```python
from build123d import *
from OCP.BRepFilletAPI import BRepFilletAPI_MakeChamfer

# Parameters (mm, degrees)
SKETCH_1_W          = 23
SKETCH_1_H          = 2
EXTRUDE_1_DEPTH     = 5
CHAMFER_1_SIZE      = 2
CHAMFER_1_SIZE2     = 1.678199262
SKETCH_2_W          = 5
SKETCH_2_H          = 2
EXTRUDE_2_DEPTH     = 14
CUT_EXTRUDE_1_DEPTH = 27.944387171
SKETCH_4_W          = 5
SKETCH_4_H          = 2
EXTRUDE_3_DEPTH     = 0.5
CHAMFER_3_SIZE      = 0.419549816
CHAMFER_3_SIZE_2    = 0.5
SKETCH_5_W          = 5
SKETCH_5_H          = 2
CUT_EXTRUDE_2_DEPTH = 19.227726134
CHAMFER_4_SIZE      = 1.5
CHAMFER_4_SIZE2     = 0.545955351
SKETCH_6_W          = 5
SKETCH_6_H          = 2
EXTRUDE_4_DEPTH     = 0.5
CHAMFER_5_SIZE      = 0.5
CHAMFER_6_SIZE      = 0.5
CHAMFER_6_SIZE2     = 1.37373871


with BuildPart() as part:
    # 草图1 → 凸台-拉伸1 (new body)
    with BuildSketch(Plane(origin=(0, 0, 0), x_dir=(1, 0, 0), z_dir=(0, 1, 0))):
        Rectangle(SKETCH_1_W, SKETCH_1_H)
    extrude(amount=EXTRUDE_1_DEPTH)

    # 倒角1
    chamfer_1_edges = [part.edges().sort_by_distance(p)[0] for p in [
        (0, 5, 1),
    ]]
    chamfer_1_side = [part.faces().sort_by_distance(p)[0] for p in [
        (0, 2.5, 1),
    ]]
    chamfer(chamfer_1_edges, length=CHAMFER_1_SIZE, length2=CHAMFER_1_SIZE2, reference=chamfer_1_side[0])

    # 草图2 → 凸台-拉伸2 (add)
    with BuildSketch(Plane(origin=(0, 0, 0), x_dir=(1, 0, 0), z_dir=(0, 1, 0))):
        with Locations((-9, 0)):
            Rectangle(SKETCH_2_W, SKETCH_2_H)
        with Locations((9, 0)):
            Rectangle(SKETCH_2_W, SKETCH_2_H)
    extrude(amount=EXTRUDE_2_DEPTH)

    # 草图3 → 切除-拉伸1 (cut, through all)
    with BuildSketch(Plane(origin=(11.5, 0, 0), x_dir=(0, 0, -1), z_dir=(1, 0, 0))):
        Polygon((-1, 1.821800738), (1, 3.5), (1, 0), (-1, 0), align=None)
    extrude(amount=-CUT_EXTRUDE_1_DEPTH, mode=Mode.SUBTRACT)

    # 草图4 → 凸台-拉伸3 (add)
    with BuildSketch(Plane(origin=(0, 0, -1), x_dir=(-1, 0, 0), z_dir=(0, 0, -1))):
        with Locations((-9, 13)):
            Rectangle(SKETCH_4_W, SKETCH_4_H)
    extrude(amount=EXTRUDE_3_DEPTH)

    # 倒角3
    chamfer_3_edges_1 = [part.edges().sort_by_distance(p)[0] for p in [
        (9, 12, -1.5),
    ]]
    chamfer_3_side_1 = [part.faces().sort_by_distance(p)[0] for p in [
        (9, 12.008390996, -1.5),
    ]]
    chamfer_3_edges_2 = [part.edges().sort_by_distance(p)[0] for p in [
        (9, 14, -1.5),
    ]]
    chamfer_3_side_2 = [part.faces().sort_by_distance(p)[0] for p in [
        (9, 13.991609004, -1.5),
    ]]
    chamfer_3 = BRepFilletAPI_MakeChamfer(part.part.solid().wrapped)
    for e in chamfer_3_edges_1:
        chamfer_3.Add(CHAMFER_3_SIZE - 0.0001, CHAMFER_3_SIZE_2 - 0.0001, e.wrapped, chamfer_3_side_1[0].wrapped)
    for e in chamfer_3_edges_2:
        chamfer_3.Add(CHAMFER_3_SIZE - 0.0001, CHAMFER_3_SIZE_2 - 0.0001, e.wrapped, chamfer_3_side_2[0].wrapped)
    add(Compound.cast(chamfer_3.Shape()), mode=Mode.REPLACE)  # a hair under: the kernel refuses the full size

    # 草图5 → 切除-拉伸2 (cut, through all)
    with BuildSketch(Plane(origin=(0, 0, -1), x_dir=(-1, 0, 0), z_dir=(0, 0, -1))):
        with Locations((9, 13)):
            Rectangle(SKETCH_5_W, SKETCH_5_H)
    extrude(amount=-CUT_EXTRUDE_2_DEPTH, mode=Mode.SUBTRACT)

    # 倒角4
    chamfer_4_edges = [part.edges().sort_by_distance(p)[0] for p in [
        (9, 14, 1),
    ]]
    chamfer_4_side = [part.faces().sort_by_distance(p)[0] for p in [
        (0, 2.082052258, 1),
    ]]
    chamfer(chamfer_4_edges, length=CHAMFER_4_SIZE, length2=CHAMFER_4_SIZE2, reference=chamfer_4_side[0])

    # 草图6 → 凸台-拉伸4 (add)
    with BuildSketch(Plane(origin=(0, 0, -1), x_dir=(-1, 0, 0), z_dir=(0, 0, -1))):
        with Locations((9, 11)):
            Rectangle(SKETCH_6_W, SKETCH_6_H)
    extrude(amount=EXTRUDE_4_DEPTH)

    # 倒角5
    chamfer_5_edges = [part.edges().sort_by_distance(p)[0] for p in [
        (-9, 10, -1),
    ]]
    chamfer(chamfer_5_edges, length=CHAMFER_5_SIZE - 0.0001)  # a hair under: the kernel refuses the full size
    chamfer_5_2_edges = [part.edges().sort_by_distance(p)[0] for p in [
        (-9, 12, -1.5),
    ]]
    chamfer(chamfer_5_2_edges, length=CHAMFER_5_SIZE)

    # 倒角6
    chamfer_6_edges = [part.edges().sort_by_distance(p)[0] for p in [
        (-9, 12, 1),
    ]]
    chamfer_6_side = [part.faces().sort_by_distance(p)[0] for p in [
        (-9, 12, 0),
    ]]
    chamfer(chamfer_6_edges, length=CHAMFER_6_SIZE, length2=CHAMFER_6_SIZE2, reference=chamfer_6_side[0])


solid = part.part
```
Geometry check sheet. Reference: the model listing, model coordinates, mm. A direction names the side the tool comes from. Round coordinates to 2 decimals unless told otherwise and drop trailing zeros. Loops run counter-clockwise (first coordinate to the right, second up) from the corner with the lowest first, then second, coordinate; pieces in that order, holes last. Notation, with made-up numbers: M -25,67.5 L -19,67.5 A15 cw -19,96.5 Z; hole C 71.5,44 d11. An arc over 180 degrees is marked long. Return JSON: item names as keys, results as strings. Group by question number.
(1) Go/stop test with flat-tipped pins: pin 1 (2.5 mm diameter, centred on x = -3, y = 6, fed in from -Z); pin 2 (0.8 mm diameter, centred on x = -9, z = -0.5, fed in from +Y); pin 3 (1.5 mm diameter, centred on x = 8.5, z = 0.5, fed in from +Y). Record where each tip stops, or that it passes through.
(2) Section check A-A, the plane y = 6.25. Enter the section's corners in (x, z), and give its area (3 significant figures).
(3) Set-up check for faces 5 (the face through (-8.965, 11.304, 0.754)), 6 (the face through (6.5, 10, 0)), 7 (the face through (2, 4, -1)): record each of +Z, -Z, +X, -X, +Y, -Y from which the full face is reachable in a straight line by a thin tool's end or side.
(4) Section check C-C, the plane z = 0.75. Enter the section's corners in (x, y), and give its area (3 significant figures).
(5) Scan lines: line 1 along X through (y, z) = (8.5, -0.75); line 2 along Z through (x, y) = (9, 5.5); line 3 along X through (y, z) = (12.75, -1.35). Record each from-to range of solid material in increasing order. Write a range as [from, to].
(6) Mould release check, pull along X, two halves, no side actions. Record for faces 1 (the face through (-9, 12, 0)), 2 (the face through (-0.09, 4.01, 0.15)), 3 (the face through (-6.5, 8, 0)), 4 (the face through (11.5, 8, 0)): pulls with the +X half, pulls with the -X half, needs draft (parallel to the pull), parting line crosses it, or undercut.
Data:
{
 "1": {"pin 1": "z = -1", "pin 2": "y = 12", "pin 3": "y = 14"},
 "2": {"outline": "M -11.5,-1 L -6.5,-1 L -6.5,1 L -11.5,1 Z; M 6.5,-1 L 11.5,-1 L 11.5,1 L 6.5,1 Z", "area": "20.0 mm²"},
 "3": {"face 5": "+Z, -X, +Y", "face 6": "+Z, +Y", "face 7": "-Z, +X, -Y"},
 "4": {"outline": "M -11.5,2.03 L 11.5,2.03 L 11.5,13.19 L 6.5,13.19 L 6.5,3.3 L -6.5,3.3 L -6.5,11.31 L -11.5,11.31 Z", "area": "119 mm²"},
 "5": {"line 1": "[-11.5, -6.5], [6.5, 11.5]", "line 2": "[-1, 1]", "line 3": "[6.5, 11.5]"},
 "6": {"face 1": "needs draft", "face 2": "undercut", "face 3": "undercut", "face 4": "pulls with the +X half"}
}
